CAD build for the part. Positions are in the model's coordinates, mm. Coordinates: 2 decimals unless noted, no trailing zeros. Answer as a JSON object with one key per item and string values. Group by question number.
from build123d import *

# Parameters (mm, degrees)
F0_W     = 670
F0_H     = 210
F1_DEPTH = 10
F2_W     = 10
F2_H     = 122.5349456072
F3_DEPTH = 25
F5_D     = 2
F5_DEPTH = 12
F5_TIP   = 0.600860619
F7_D     = 2
F7_DEPTH = 12
F7_TIP   = 0.600860619


with BuildPart() as f1:
    # F0 (on Top) → F1 (new body)
    with BuildSketch(Plane.XY):
        with Locations((-335, 105)):
            Rectangle(F0_W, F0_H)
    extrude(amount=F1_DEPTH)

    # F2 (on face) → F3 (cut)
    with BuildSketch(Plane.XY.offset(10)):
        with Locations((-590, 61.2674728036)):
            Rectangle(F2_W, F2_H)
        with Locations((-505, 61.2674728036)):
            Rectangle(F2_W, F2_H)
        with Locations((-420, 61.2674728036)):
            Rectangle(F2_W, F2_H)
        with Locations((-335, 61.2674728036)):
            Rectangle(F2_W, F2_H)
        with Locations((-250, 61.2674728036)):
            Rectangle(F2_W, F2_H)
        with Locations((-165, 61.2674728036)):
            Rectangle(F2_W, F2_H)
        with Locations((-80, 61.2674728036)):
            Rectangle(F2_W, F2_H)
    extrude(amount=-F3_DEPTH, mode=Mode.SUBTRACT)

    # F5
    with Locations(Plane(origin=(-670, 0, 0), x_dir=(0, -1, 0), z_dir=(-1, 0, 0))):
        with Locations((-190, 5), (-20, 5)):
            Hole(F5_D / 2, depth=F5_DEPTH)
            with Locations((0, 0, -(F5_DEPTH + F5_TIP / 2))):  # 118° drill point
                Cone(0, F5_D / 2, F5_TIP, mode=Mode.SUBTRACT)

    # F7
    with Locations(Plane.YZ):
        with Locations((20, 5), (190, 5)):
            Hole(F7_D / 2, depth=F7_DEPTH)
            with Locations((0, 0, -(F7_DEPTH + F7_TIP / 2))):  # 118° drill point
                Cone(0, F7_D / 2, F7_TIP, mode=Mode.SUBTRACT)


solid = f1.part
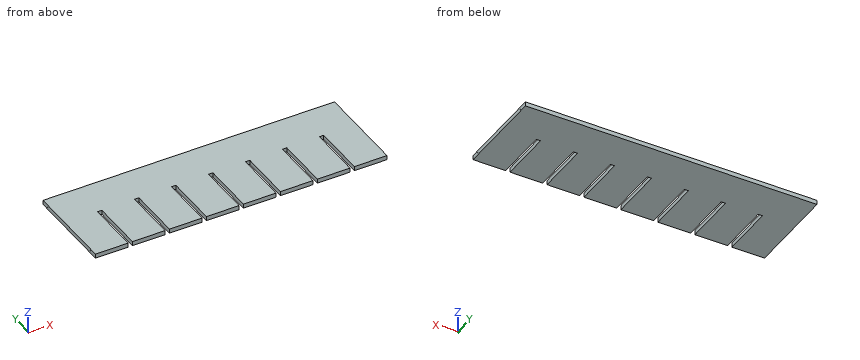
Item 1: Drill centre lines: L1, parallel to Y at x = -661, z = 5; L2, parallel to Z at x = -665.5, y = 190. Where is each one in solid material? Low to high.
Item 2: Band-saw the part on A-A, the plane y = 56.5. Count the separate pieces of the cut face and the enclosed holes in it, and give its area (3 significant figures).
Item 3: Flat gauge pins, fed straight in: P1, Ø1.8, axis at y = 190, z = 5, coming from the +X side; P2, Ø5, axis at x = -163.5, z = 3.5, coming from the -Y side; P3, Ø1.8, axis at y = 190, z = 5, coming from the -X side. Where does each tip first touch, or does it go through?
Reply:
{
 "1": {"L1": "0 to 19, 21 to 189, 191 to 210", "L2": "0 to 4, 6 to 10"},
 "2": {"separate pieces": "8", "enclosed holes": "0", "area": "6,000 mm²"},
 "3": {"P1": "x = -12.06", "P2": "y = 122.53", "P3": "x = -657.94"}
}
